Design review of the part built by this model. Coordinates are the model's own, in mm. A direction names the side the tool comes from. Round coordinates to 2 decimals unless told otherwise and drop trailing zeros. Write each loop counter-clockwise with the first axis right and the second up, starting at its lowest first coordinate (ties: lowest second). Pieces come first, ordered by that corner, then holes. Notation, with made-up numbers: M -9.5,-22.75 L 8.5,-22.75 A14 ccw 8.5,-13.75 Z; hole C 9,81.25 d7. An arc over 180 degrees is marked long. Use CSV: the item, a comma, the result in double quotes.
from build123d import *

# Parameters (mm, degrees)
CROQUIS1_W              = 200
CROQUIS1_H              = 200
SALIENTE_EXTRUIR1_DEPTH = 100
CROQUIS2_W              = 194
CROQUIS2_H              = 187
CORTAR_EXTRUIR1_DEPTH   = 97
REDONDEO2_R             = 4.5
CROQUIS3_R              = 1.6
CROQUIS3_W              = 8
CROQUIS3_H              = 3
CORTAR_EXTRUIR2_DEPTH   = 10
CORTAR_EXTRUIR3_REACH   = 202
CROQUIS4_R              = 10
CROQUIS5_R              = 1.6
CORTAR_EXTRUIR4_DEPTH   = 4


with BuildPart() as part:
    # Croquis1 → Saliente-Extruir1 (new body)
    with BuildSketch(Plane(origin=(0, 0, 0), x_dir=(1, 0, 0), z_dir=(0, 1, 0))):
        Rectangle(CROQUIS1_W, CROQUIS1_H)
    extrude(amount=SALIENTE_EXTRUIR1_DEPTH)

    # Croquis2 → Cortar-Extruir1 (cut)
    with BuildSketch(Plane(origin=(0, 100, 0), x_dir=(1, 0, 0), z_dir=(0, 1, 0))):
        with Locations((0, 3.5)):
            Rectangle(CROQUIS2_W, CROQUIS2_H)
    extrude(amount=-CORTAR_EXTRUIR1_DEPTH, mode=Mode.SUBTRACT)

    # Redondeo2
    redondeo2_edges = [part.edges().sort_by_distance(p)[0] for p in [
        (-97, 51.5, 90),
        (-97, 51.5, -97),
        (97, 51.5, -97),
        (97, 51.5, 90),
        (-97, 3, -3.5),
        (0, 3, -97),
        (97, 3, -3.5),
        (0, 3, 90),
    ]]
    fillet(redondeo2_edges, radius=REDONDEO2_R)

    # Croquis3 → Cortar-Extruir2 (cut)
    with BuildSketch(Plane.XY.offset(100)):
        with Locations((-70, 70)):
            Circle(CROQUIS3_R)
        with Locations((-41, 70)):
            Circle(CROQUIS3_R)
        with Locations((-70.5, 94.5)):
            Rectangle(CROQUIS3_W, CROQUIS3_H)
        with Locations((-41, 94.5)):
            Rectangle(CROQUIS3_W, CROQUIS3_H)
    cortar_extruir2 = extrude(amount=-CORTAR_EXTRUIR2_DEPTH, mode=Mode.SUBTRACT)

    # Simetría1: Cortar-Extruir2 across plane
    add(cortar_extruir2.mirror(Plane(origin=(0, 0, 0), x_dir=(0, 0, 1), z_dir=(1, 0, 0))), mode=Mode.SUBTRACT)

    # Croquis4 → Cortar-Extruir3 (cut, up to next)
    with BuildSketch(Plane.XY.offset(100), mode=Mode.PRIVATE) as cortar_extruir3_sk1:
        with Locations((60, 15)):
            Circle(CROQUIS4_R)
    cortar_extruir3_tool1 = extrude(cortar_extruir3_sk1.sketch, amount=-CORTAR_EXTRUIR3_REACH, mode=Mode.PRIVATE) & part.part
    add(cortar_extruir3_tool1.solids().sort_by_distance((60, 15, 100))[0], mode=Mode.SUBTRACT)

    # Croquis5 → Cortar-Extruir4 (cut)
    with BuildSketch(Plane(origin=(0, 100, 0), x_dir=(1, 0, 0), z_dir=(0, 1, 0))):
        with Locations((-70, -95.159266914)):
            Circle(CROQUIS5_R)
        with Locations((-41, -95.159266914)):
            Circle(CROQUIS5_R)
    cortar_extruir4 = extrude(amount=-CORTAR_EXTRUIR4_DEPTH, mode=Mode.SUBTRACT)

    # Simetría2: Cortar-Extruir4 across plane
    add(cortar_extruir4.mirror(Plane(origin=(0, 0, 0), x_dir=(0, 0, 1), z_dir=(1, 0, 0))), mode=Mode.SUBTRACT)


solid = part.part
1) Add section D-D on z = -29. Write out the cut boundary in (x, y).
Answers:
outline,"M -100,0 L 100,0 L 100,100 L 97,100 L 97,7.5 A4.5 cw 92.5,3 L -92.5,3 A4.5 cw -97,7.5 L -97,100 L -100,100 Z"
2) The part is to be moulded in two halves that separate along Y. For faces 1 (the face through (-1, 0, -1)), 2 (the face through (-41, 93, 95)), 3 (the face through (-1, 54, 90)), say which applies: released by +Y, released by -Y, zero draft, split by the parting line, or undercut.
Answers:
face 1,"released by -Y"
face 2,"undercut"
face 3,"zero draft"
3) For pin 1 Ø3 at (x, z) = (-18, 52) entering from -Y; pin 2 Ø5 at (x, z) = (-37.5, -27) entering from +Y, all flat-tipped, find the tip position at first contact; note any pin that passes through.
Answers:
pin 1,"y = 0"
pin 2,"y = 3"
4) Machinability: for faces 4 (the face through (-71, 93, 95)), 5 (the face through (100, 49, 1)), 6 (the face through (-1, 3, -5)), which of the approach directions +Z, -Z, +X, -X, +Y, -Y give a long, thin tool a straight path to every point of the face, cutting with its end or side? Answer none if there is none.
Answers:
face 4,"+Z"
face 5,"+Z, -Z, +X, +Y, -Y"
face 6,"+Y"
5) Add section C-C on y = 78. Write out the cut boundary in (x, z), then the cut area to 3 significant figures.
Answers:
outline,"M -100,-100 L 100,-100 L 100,100 L -100,100 Z; hole M -97,-92.5 A4.5 ccw -92.5,-97 L 92.5,-97 A4.5 ccw 97,-92.5 L 97,85.5 A4.5 ccw 92.5,90 L -92.5,90 A4.5 ccw -97,85.5 Z"
area,"3,740 mm²"
6) Wall thickness on line 1 along Y through (x, z) = (-41, 93); line 2 along Z through (x, y) = (41, 97); line 3 along Z through (x, y) = (33, 82): over which ranges is each line inside the solid? List them lowest first. Write a range as [from, to].
Answers:
line 1,"[0, 68.4], [71.6, 93], [96, 100]"
line 2,"[-100, -97], [90, 93.56], [96.76, 100]"
line 3,"[-100, -97], [90, 100]"
7) Add section A-A on x = 60. Write out the cut boundary in (y, z).
Answers:
outline,"M 0,-100 L 100,-100 L 100,-97 L 7.5,-97 A4.5 cw 3,-92.5 L 3,85.5 A4.5 cw 5,89.24 L 5,100 L 0,100 Z; M 25,90 L 100,90 L 100,100 L 25,100 Z"
8) Add section B-B on y = 15. Write out the cut boundary in (x, z), then the cut area to 3 significant figures.
Answers:
outline,"M -100,-100 L 100,-100 L 100,100 L 70,100 L 70,90 L 92.5,90 A4.5 cw 97,85.5 L 97,-92.5 A4.5 cw 92.5,-97 L -92.5,-97 A4.5 cw -97,-92.5 L -97,85.5 A4.5 cw -92.5,90 L 50,90 L 50,100 L -100,100 Z"
area,"3,540 mm²"
